```python
from build123d import *

# Parameters (mm, degrees)
SKETCH1_W           = 50.8
SKETCH1_H           = 19.05
SKETCH1_R           = 2
BOSS_EXTRUDE1_DEPTH = 12.7
SKETCH2_W           = 9.525
SKETCH2_H           = 6.35
CUT_EXTRUDE1_DEPTH  = 10.5
FILLET1_R           = 4.7625
FILLET2_R           = 4.7625


with BuildPart() as part:
    # Sketch1 → Boss-Extrude1 (new body)
    with BuildSketch(Plane.XY):
        with Locations((25.4, 9.525)):
            Rectangle(SKETCH1_W, SKETCH1_H)
        with Locations((3.81, 3.81)):
            Circle(SKETCH1_R, mode=Mode.SUBTRACT)
        with Locations((3.81, 15.24)):
            Circle(SKETCH1_R, mode=Mode.SUBTRACT)
    extrude(amount=BOSS_EXTRUDE1_DEPTH)

    # Sketch2 → Cut-Extrude1 (cut)
    with BuildSketch(Plane(origin=(0, 19.05, 0), x_dir=(1, 0, 0), z_dir=(0, 1, 0))):
        with Locations((4.7625, -6.35)):
            Rectangle(SKETCH2_W, SKETCH2_H)
    extrude(amount=-CUT_EXTRUDE1_DEPTH, mode=Mode.SUBTRACT)

    # Fillet1
    fillet1_edges = [part.edges().sort_by_distance(p)[0] for p in [
        (9.525, 8.55, 6.35),
    ]]
    fillet(fillet1_edges, radius=FILLET1_R)

    # Fillet2
    fillet2_edges = [part.edges().sort_by_distance(p)[0] for p in [
        (0, 19.05, 1.5875),
        (0, 19.05, 11.1125),
        (0, 0, 6.35),
    ]]
    fillet(fillet2_edges, radius=FILLET2_R)


solid = part.part
```
Source: CAD feature listing. Evaluate the final solid. Frame: model axes, mm. A direction names the side the tool comes from. Round coordinates to 2 decimals unless told otherwise and drop trailing zeros. Write each loop counter-clockwise with the first axis right and the second up, starting at its lowest first coordinate (ties: lowest second). Pieces come first, ordered by that corner, then holes. Notation, with made-up numbers: M 18.5,7.25 L 49.5,7.25 A31 cw 49.5,43.25 Z; hole C 59,30 d7. An arc over 180 degrees is marked long. Use CSV: the item, a comma, the result in double quotes. Start each with the question number.
Q1. Cut plane B-B on y = 3.81. Output: boundary loops of the cut face in (x, z), plus the area to 3 significant figures.
Q2. Line query: line 1 (Y direction, x = 3.81, z = 10.75); line 2 (X direction, y = 16, z = 8) (3 decimals); line 3 (Z direction, x = 7, y = 9.75) (3 decimals). Output: solid intervals per line, ascending. Write a range as from..to.
Q3. Cut plane C-C on x = 3.81. Output: boundary loops of the cut face in (y, z) (3 decimals), plus the area to 3 significant figures.
Q4. First-contact query: P1, Ø5, axis at x = 3, z = 7.5, coming from the +Y side; P2, Ø1.7, axis at y = 15, z = 6.5, coming from the -X side (3 decimals). Flat tips, straight axial feed; report the tip coordinate or a pass-through.
Q5. Cut plane A-A on z = 10.25. Count the separate pieces of the cut face and the enclosed holes in it, plus the area to 3 significant figures.
Q6. Pull-direction query (Z, two-part tool) for faces 1 (the face through (25, 10, 0)), 2 (the face through (5, 13, 3.175)), 3 (the face through (27, 0, 6)), 4 (the face through (9.525, 16, 6)); classes: +Z half, -Z half, draft (parallel to the pull), parting line (faces both ways), or undercut.
Q7. Cut plane D-D on y = 14.75. Output: boundary loops of the cut face in (x, z) (3 decimals).
Q8. Access query for faces 5 (the face through (8.093, 9.908, 6.306)), 6 (the face through (0, 8, 6)). Directions: +Z, -Z, +X, -X, +Y, -Y. A direction counts if a zero-diameter tool reaches every point of the face in a straight line with its end or side. Return the directions, or none.
Results found:
1,outline,"M 0.1,0 L 1.81,0 L 1.81,12.7 L 0.1,12.7 Z; M 5.81,0 L 50.8,0 L 50.8,12.7 L 5.81,12.7 Z"
1,area,"593 mm^2"
2,line 1,"0.1..1.81, 5.81..13.24, 17.24..18.95"
2,line 2,"9.525..50.8"
2,line 3,"0..3.175, 9.525..12.7"
3,outline,"M 0.096,0 L 1.81,0 L 1.81,12.7 L 0.096,12.7 Z; M 5.81,0 L 13.24,0 L 13.24,3.175 L 8.55,3.175 L 8.55,9.525 L 13.24,9.525 L 13.24,12.7 L 5.81,12.7 Z; M 17.24,0 L 18.954,0 L 18.954,3.175 L 17.24,3.175 Z; M 17.24,9.525 L 18.954,9.525 L 18.954,12.7 L 17.24,12.7 Z"
3,area,"97.2 mm^2"
4,P1,"y = 19.04"
4,P2,"x = 9.525"
5,separate pieces,"1"
5,enclosed holes,"2"
5,area,"933 mm^2"
6,face 1,"-Z half"
6,face 2,"undercut"
6,face 3,"draft"
6,face 4,"undercut"
7,outline,"M 0.023,0 L 1.871,0 L 1.871,3.175 L 0.023,3.175 Z; M 0.023,9.525 L 1.871,9.525 L 1.871,12.7 L 0.023,12.7 Z; M 5.749,0 L 50.8,0 L 50.8,12.7 L 5.749,12.7 L 5.749,9.525 L 9.525,9.525 L 9.525,3.175 L 5.749,3.175 Z"
8,face 5,"-X, +Y"
8,face 6,"+Z, -Z, -X, +Y, -Y"
